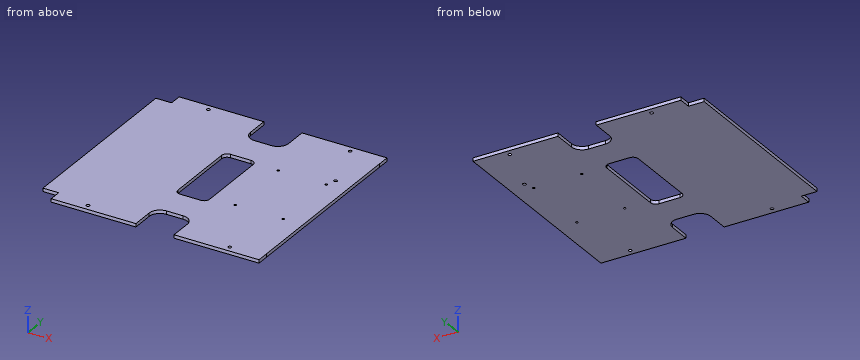
Autodesk Inventor part; units mm, degrees
ref_plane "РабПлоскость1" through (199.2972, 37.5, 4) normal (0, 1, 0) x (1, 0, 0)
ref_plane "YZ Plane" through (0, 0, 0) normal (1, 0, 0) x (0, 1, 0)
ref_plane "XZ Plane" through (0, 0, 0) normal (0, 1, 0) x (-1, 0, 0)
sketch "Эскиз1" plane through (0, 0, 0) normal (0, 0, 1) x (1, 0, 0)
  circle A0 centre (25, 157.5) radius 2
  circle A1 centre (196.5682, 157.5) radius 2
  line L0 (236.5682, 150) -> (236.5682, 165)
  line L1 (-34.0192, 150) -> (-15, 150)
  line L2 (-34.0192, 150) -> (-15, 150)
  line L3 (-34.0192, 37.5) -> (-34.0192, 150)
  line L4 (236.5682, 165) -> (-15, 165)
  line L5 (236.5682, 37.5) -> (236.5682, 165)
  line L6 (-34.0192, 37.5) -> (236.5682, 37.5)
  line L7 (-15, 165) -> (-15, 150)
  dimension "d5" = 127.5
  dimension "d6" = 7.5
  dimension "d7" = 7.5
  dimension "d9" = 15
extrude "Выдавливание1" add sketch "Эскиз1" along normal blind 4
sketch "Эскиз2" plane through (0, 0, 4) normal (0, 0, 1) x (1, 0, 0)
  line L0 (236.5682, 150) -> (199.2972, 150)
  line L1 (-15, 150) -> (-34.0192, 150)
  line L2 (-34.0192, 37.5) -> (236.5682, 37.5)
  line L3 (199.2972, 150) -> (236.5682, 150)
  line L4 (236.5682, 150) -> (236.5682, 37.5)
  line L5 (236.5682, 37.5) -> (199.2972, 37.5)
  line L6 (199.2972, 37.5) -> (199.2972, 150)
  point P0 (0, 0)
  point P1 (-24.5096, 150)
  point P2 (-15, -15)
extrude "Выдавливание2" cut sketch "Эскиз2" against normal blind 4
mirror "Зеркальное отражение2" about plane through (-34.0192, 37.5, 0) normal (0, -1, 0) of "Выдавливание1", "Выдавливание2"
sketch "Эскиз3" plane through (0, 0, 4) normal (0, 0, 1) x (1, 0, 0)
  line L0 (236.5682, -90) -> (-15, -90)
  line L1 (87.4676, -90) -> (133.662, -90)
  line L2 (133.662, -90) -> (133.662, -50.4003)
  line L3 (133.662, -50.4003) -> (87.4676, -50.4003)
  line L4 (87.4676, -50.4003) -> (87.4676, -90)
  point P0 (0, 0)
extrude "Выдавливание3" cut sketch "Эскиз3" against normal blind 10
ref_plane "РабПлоскость1" through (199.2972, 37.5, 4) normal (0, 1, 0) x (1, 0, 0)
mirror "Зеркальное отражение3" about plane through (199.2972, 37.5, 4) normal (0, 1, 0) of "Выдавливание3"
move faces "Перенос1" translate (37.25, 0, 0) faces at (199.2972, 0, 2.6667)
sketch "Эскиз4" plane through (0, 0, 4) normal (0, 0, 1) x (1, 0, 0)
  circle A0 centre (154.5472, 83.5) radius 1.375
  circle A1 centre (154.5472, -2.5) radius 1.375
  circle A2 centre (212.5472, -2.5) radius 1.375
  circle A3 centre (212.5472, 83.5) radius 1.375
  circle A4 centre (216.5472, 95.5) radius 2
  circle A5 centre (216.5472, -20.5) radius 2
  line L0 (215.9472, 87.5) -> (138.1472, 87.5)
  line L1 (138.1472, -12.5) -> (215.9472, -12.5)
  line L2 (125.662, 87.5) -> (87.4676, 87.5)
  line L3 (87.4676, 87.5) -> (87.4676, -12.5)
  line L4 (87.4676, -12.5) -> (125.662, -12.5)
  line L5 (125.662, -12.5) -> (125.662, 87.5)
  line L6 (87.4676, -90) -> (87.4676, -50.4003)
  line L7 (133.662, -50.4003) -> (133.662, -90)
  point P0 (0, 0)
  dimension "d15" = 8
extrude "Выдавливание4" cut sketch "Эскиз4" against normal blind 10 contours A0 | A1 | A2 | A3 | A4 | L5 L4 L3 L2
fillet "Сопряжение1" radius 13 4 edges at (87.4676, 125.4003, 2) (133.662, 125.4003, 2) (87.4676, -50.4003, 2) (133.662, -50.4003, 2)
fillet "Сопряжение2" radius 6.5 4 edges at (87.4676, -12.5, 2) (125.662, -12.5, 2) (87.4676, 87.5, 2) (125.662, 87.5, 2)
properties part number "KB33-046-004-018 - Полка электроники"
The model under review builds one solid part; all positions refer to its coordinate system, in mm. Coordinates: 2 decimals unless noted, no trailing zeros. One line per question, with ' | ' between items.
(1) For probe 1 along X at (y, z) = (-82.5, 2.05); probe 2 along Y at (x, z) = (102, 2.9); probe 3 along X at (y, z) = (-62.5, 1.7), list the stretches that pass through material, from the lowest coordinate up. Write a range as from..to.
Geometry results:
probe 1: x = -15..23, 27..87.47, 133.66..194.57, 198.57..236.57 | probe 2: y = -50.4..-12.5, 87.5..125.4 | probe 3: x = -34.02..87.5, 133.63..236.55
(2) Insertion check: pin 1 (2 mm diameter, centred on x = -20.5, z = 3, fed in from -Y); pin 2 (1.2 mm diameter, centred on x = 107.5, z = 1, fed in from +Y); pin 3 (3 mm diameter, centred on x = 216.55, y = 95.5, fed in from +Z); pin 4 (1.2 mm diameter, centred on y = -78, z = 2, fed in from -X). Each pin has a flat end and moves straight along its axis. Give the tip position at first contact, or say it passes through.
Geometry results:
pin 1: stops at y = -75 | pin 2: stops at y = 125.4 | pin 3: passes through | pin 4: stops at x = -15
(3) Add section A-A, the plane z = 2.85. State how many separate pieces and enclosed holes the cut face has, then the cut area to 3 significant figures.
Geometry results:
separate pieces: 1 | enclosed holes: 10 | area: 61,000 mm²
